```python
from build123d import *

# Parameters (mm, degrees)
F0_W            = 42.7
F0_H            = 30.1
F0_R            = 2
F1_DEPTH        = 2
F2_DEPTH        = 3
F3_DEPTH        = 0.1
F4_DEPTH        = 0.1
F6_W            = 1.7407113919
F6_H            = 30.1
F7_DEPTH        = 6.5
F9_W            = 1.7492394143
F9_H            = 30.1
F10_DEPTH       = 5
F11_D           = 2
F11_CSINK_D     = 4
F11_CSINK_ANGLE = 90
F12_D           = 7.59


# Not quite as in the source:
# - a feature names something its author has since deleted; it is built from what else it names


with BuildPart() as f1:
    # F0 (on Front) → F1 (new body)
    with BuildSketch(Plane.XZ):
        Rectangle(F0_W, F0_H)
        with Locations((-17.35, 0)):
            Circle(F0_R, mode=Mode.SUBTRACT)
        with Locations((15.29, -12.86)):
            Circle(F0_R, mode=Mode.SUBTRACT)
        with Locations((18.83, 12.5)):
            Circle(F0_R, mode=Mode.SUBTRACT)
        with Locations((18.83, 12.5)):
            Circle(F0_R)
        with Locations((-17.35, 0)):
            Circle(F0_R)
        with Locations((15.29, -12.86)):
            Circle(F0_R)
    extrude(amount=-F1_DEPTH)

    # F0 (on Front) → F2 (join)
    with BuildSketch(Plane.XZ):
        with Locations((18.83, 12.5)):
            Circle(F0_R)
        with Locations((15.29, -12.86)):
            Circle(F0_R)
        with Locations((-17.35, 0)):
            Circle(F0_R)
    extrude(amount=-F2_DEPTH)

    # F3 (add): a face of the model
    f3_faces = [f1.faces().sort_by_distance(p)[0] for p in [
        (-21.35, 1, 0),
    ]]
    extrude(f3_faces, amount=F3_DEPTH)

    # F4 (add): a face of the model
    f4_faces = [f1.faces().sort_by_distance(p)[0] for p in [
        (21.35, 1, 0),
    ]]
    extrude(f4_faces, amount=F4_DEPTH)

    # F6 (on face) → F7 (join)
    with BuildSketch(Plane(origin=(-16.2487833534, 9.1931193, 0), x_dir=(0.4924235601, 0.8703556959, 0), z_dir=(0.8703556959, -0.4924235601, 0))):
        with Locations((-9.6921296683, 0)):
            Rectangle(F6_W, F6_H)
    extrude(amount=-F7_DEPTH)

    # F9 (on face) → F10 (join)
    with BuildSketch(Plane(origin=(16.4083841089, 9.0953158313, 0), x_dir=(0.4848096202, -0.8746197071, 0), z_dir=(-0.8746197071, -0.4848096202, 0))):
        with Locations((9.5245466471, 0)):
            Rectangle(F9_W, F9_H)
    extrude(amount=-F10_DEPTH)

    # F11 (through all)
    with Locations(Plane.XZ):
        with Locations((-17.35, 0), (18.83, 12.5), (15.29, -12.86)):
            CounterSinkHole(F11_D / 2, F11_CSINK_D / 2, counter_sink_angle=F11_CSINK_ANGLE)

    # F12 (through all)
    with Locations(Plane.XZ):
        with Locations((-17.255, 7.655), (-17.255, -7.695)):
            Hole(F12_D / 2)


solid = f1.part
```
For this review, take the finished solid that the model builds, in its own axes (mm). A direction names the side the tool comes from. Round coordinates to 2 decimals unless told otherwise and drop trailing zeros. Write each loop counter-clockwise with the first axis right and the second up, starting at its lowest first coordinate (ties: lowest second). Pieces come first, ordered by that corner, then holes. Notation, with made-up numbers: (17.5, 77.25) - (24.5, 77.25) arc R16 ccw to (24.5, 89.25) - close; hole circle Ø4 at (-13.5, 4.25). An arc over 180 degrees is marked (long way). Use CSV: the item, a comma, the result in double quotes.
1) For faces 4 (the cylindrical face through (19.62, 2.01, 11.89)), 5 (the cylindrical face through (13.703, 2.493, -14.077)), 6 (the flat face through (23.188, 2.963, -0.211)), list the 3-axis set-ups (+Z, -Z, +X, -X, +Y, -Y) from which the entire face can be reached by the end or side of a thin tool; tool diameter is ignored.
Conclusion:
face 4,"+Y, -Y"
face 5,"+Y"
face 6,"+Z, -Z, +Y"
2) Add section A-A on x = 18.83. Write out the cut boundary in (y, z), and give its area (3 significant figures).
Conclusion:
outline,"(0, -15.05) - (2, -15.05) - (2, 10.5) - (3, 10.5) - (3, 11.5) - (1, 11.5) - (0, 10.5) - close; (0, 14.5) - (1, 13.5) - (3, 13.5) - (3, 14.5) - (2, 14.5) - (2, 15.05) - (0, 15.05) - close"
area,"57.2 mm^2"
3) Add section B-B on z = -10. Write out the cut boundary in (x, y).
Conclusion:
outline,"(-27.11, 3.2) - (-21.45, 0) - (-20.27, 0) - (-20.27, 2) - (-21.45, 2) - (-26.25, 4.72) - close; (-14.24, 0) - (21.45, 0) - (25.82, 2.42) - (24.98, 3.95) - (21.45, 2) - (-14.24, 2) - close"
4) Add section C-C on x = -17.35. Write out the cut boundary in (y, z).
Conclusion:
outline,"(0, -15.05) - (2, -15.05) - (2, -11.49) - (0, -11.49) - close; (0, -3.9) - (2, -3.9) - (2, -2) - (3, -2) - (3, -1) - (1, -1) - (0, -2) - close; (0, 2) - (1, 1) - (3, 1) - (3, 2) - (2, 2) - (2, 3.86) - (0, 3.86) - close; (0, 11.45) - (2, 11.45) - (2, 15.05) - (0, 15.05) - close"
5) Wall thickness on line 1 along Z through (x, y) = (-17.35, 1.8); line 2 along Z through (x, y) = (-20, 0.55); line 3 along Z through (x, y) = (15.29, 2.45): over which ranges is each line inside the solid? List them lowest first. Write a range as from..to.
Conclusion:
line 1,"z = -15.05..-11.49, -3.9..-1, 1..3.86, 11.45..15.05"
line 2,"z = -15.05..-10.32, -5.07..5.03, 10.28..15.05"
line 3,"z = -14.86..-13.86, -11.86..-10.86"
6) Clearance check with flat-ended pins moving along their axes: pin 1 Ø10 at (x, z) = (-17.255, 7.655) entering from +Y; pin 2 Ø3 at (x, z) = (-18.5, 0) entering from +Y; pin 3 Ø3 at (x, z) = (-17.35, 0) entering from -Y; pin 4 Ø4.5 at (x, z) = (-17.255, -7.695) entering from -Y. State where each tip first meets the part, or that it passes through.
Conclusion:
pin 1,"stops at y = 2.46"
pin 2,"stops at y = 3"
pin 3,"stops at y = 0.5"
pin 4,"passes through"
7) The part is to be moulded in two halves that separate along Z. For faces 1 (the cylindrical face through (-15.442, 2.493, 0.601)), 2 (the cylindrical face through (-18.274, 2.014, -0.383)), 3 (the flat face through (14, 3, -13)), say which applies: pulls with the +Z half, pulls with the -Z half, needs draft (parallel to the pull), parting line crosses it, or undercut.
Conclusion:
face 1,"parting line crosses it"
face 2,"undercut"
face 3,"needs draft"
8) Add section D-D on z = -5. Write out the cut boundary in (x, y), and give its area (3 significant figures).
Conclusion:
outline,"(-27.11, 3.2) - (-21.45, 0) - (-19.93, 0) - (-19.93, 2) - (-21.45, 2) - (-26.25, 4.72) - close; (-14.58, 0) - (21.45, 0) - (25.82, 2.42) - (24.98, 3.95) - (21.45, 2) - (-14.58, 2) - close"
area,"93.5 mm^2"
